```python
from build123d import *

# Parameters (mm, degrees)
SKETCH1_W           = 55.5
SKETCH1_H           = 55.5
SKETCH1_R           = 1.5
SKETCH1_W_2         = 34.5
SKETCH1_H_2         = 34.5
BOSS_EXTRUDE2_DEPTH = 2
SKETCH2_W           = 67.5
SKETCH2_H           = 67.5
SKETCH2_R           = 1.5
SKETCH2_W_2         = 55.5
SKETCH2_H_2         = 55.5
BOSS_EXTRUDE5_DEPTH = 2
SKETCH3_W           = 7
SKETCH3_H           = 7
SKETCH3_R           = 1.5
BOSS_EXTRUDE6_DEPTH = 25


with BuildPart() as part:
    # Sketch1 → Boss-Extrude2 (new body)
    with BuildSketch(Plane(origin=(0, 0, 0), x_dir=(1, 0, 0), z_dir=(0, 1, 0))):
        Rectangle(SKETCH1_W, SKETCH1_H)
        with Locations(Location((21.5, -21.5, 0), (0, 0, 270))):
            Circle(SKETCH1_R, mode=Mode.SUBTRACT)
        with Locations(Location((-21.5, -21.5, 0), (0, 0, 270))):
            Circle(SKETCH1_R, mode=Mode.SUBTRACT)
        with Locations(Location((21.5, 21.5, 0), (0, 0, 270))):
            Circle(SKETCH1_R, mode=Mode.SUBTRACT)
        with Locations(Location((-21.5, 21.5, 0), (0, 0, 270))):
            Circle(SKETCH1_R, mode=Mode.SUBTRACT)
        Rectangle(SKETCH1_W_2, SKETCH1_H_2, mode=Mode.SUBTRACT)
    extrude(amount=BOSS_EXTRUDE2_DEPTH)

    # Sketch2 → Boss-Extrude5 (add)
    with BuildSketch(Plane(origin=(0, 0, 0), x_dir=(1, 0, 0), z_dir=(0, 1, 0))):
        Rectangle(SKETCH2_W, SKETCH2_H)
        with Locations(Location((-30.25, 30.25, 0), (0, 0, 270))):
            Circle(SKETCH2_R, mode=Mode.SUBTRACT)
        with Locations(Location((30.25, 30.25, 0), (0, 0, 90))):
            Circle(SKETCH2_R, mode=Mode.SUBTRACT)
        with Locations(Location((30.25, -30.25, 0), (0, 0, 270))):
            Circle(SKETCH2_R, mode=Mode.SUBTRACT)
        with Locations(Location((-30.25, -30.25, 0), (0, 0, 90))):
            Circle(SKETCH2_R, mode=Mode.SUBTRACT)
        Rectangle(SKETCH2_W_2, SKETCH2_H_2, mode=Mode.SUBTRACT)
    extrude(amount=BOSS_EXTRUDE5_DEPTH)

    # Sketch3 → Boss-Extrude6 (add)
    # profile 1 of 4: a face of its own
    with BuildSketch(Plane(origin=(0, 0, 0), x_dir=(1, 0, 0), z_dir=(0, 1, 0))):
        with Locations((-30.25, -30.25)):
            Rectangle(SKETCH3_W, SKETCH3_H)
        with Locations(Location((-30.25, -30.25, 0), (0, 0, 90))):
            Circle(SKETCH3_R, mode=Mode.SUBTRACT)
    # profile 2 of 4: a face of its own
    with BuildSketch(Plane(origin=(0, 0, 0), x_dir=(1, 0, 0), z_dir=(0, 1, 0))):
        with Locations((30.25, -30.25)):
            Rectangle(SKETCH3_W, SKETCH3_H)
        with Locations(Location((30.25, -30.25, 0), (0, 0, 270))):
            Circle(SKETCH3_R, mode=Mode.SUBTRACT)
    # profile 3 of 4: a face of its own
    with BuildSketch(Plane(origin=(0, 0, 0), x_dir=(1, 0, 0), z_dir=(0, 1, 0))):
        with Locations((-30.25, 30.25)):
            Rectangle(SKETCH3_W, SKETCH3_H)
        with Locations(Location((-30.25, 30.25, 0), (0, 0, 270))):
            Circle(SKETCH3_R, mode=Mode.SUBTRACT)
    # profile 4 of 4: a face of its own
    with BuildSketch(Plane(origin=(0, 0, 0), x_dir=(1, 0, 0), z_dir=(0, 1, 0))):
        with Locations((30.25, 30.25)):
            Rectangle(SKETCH3_W, SKETCH3_H)
        with Locations(Location((30.25, 30.25, 0), (0, 0, 90))):
            Circle(SKETCH3_R, mode=Mode.SUBTRACT)
    extrude(amount=BOSS_EXTRUDE6_DEPTH)


solid = part.part
```
Geometry check sheet. Reference: the model listing, model coordinates, mm. A direction names the side the tool comes from. Round coordinates to 2 decimals unless told otherwise and drop trailing zeros. Loops run counter-clockwise (first coordinate to the right, second up) from the corner with the lowest first, then second, coordinate; pieces in that order, holes last. Notation, with made-up numbers: (39.25, 58.5) - (75.25, 58.5) arc R12 ccw to (75.25, 81.5) - close; hole circle Ø6 at (41.25, -3.5). An arc over 180 degrees is marked (long way). Write item = value, one per line. Start each with the question number.
1. Section check D-D on z = -5.5. Enter the section's corners in (x, y).
2. Set-up check for faces 1 (the face through (30, 13, 26.75)), 2 (the face through (26.75, 13, 30)), 3 (the face through (-30.3, 25, 28.6)), 4 (the face through (-17.25, 1, 0)): record each of +Z, -Z, +X, -X, +Y, -Y from which the full face is reachable in a straight line by a thin tool's end or side.
3. Thickness scan on line 1 (X direction, y = 8.75, z = 30.25); line 2 (X direction, y = 0.85, z = -21.5); line 3 (X direction, y = 14.25, z = 28.5). Record the ranges inside material, lowest first.
4. Depth check by flat-ended pin: pin 1 (3 mm diameter, centred on x = -25, y = 22, fed in from +Z); pin 2 (3 mm diameter, centred on x = -24.5, z = -4.5, fed in from +Y). Enter the tip coordinate at first touch or a pass-through.
5. Section check C-C on x = 9.5. Enter the section's corners in (y, z), then the cut area to 3 significant figures.
6. Section check B-B on z = -21.5. Enter the section's corners in (x, y).
7. Section check A-A on y = 21.75. Enter the section's corners in (x, z), then the cut area to 3 significant figures.
8. Mould release check, pull along X, two halves, no side actions. Record for faces 5 (the face through (0, 0, -23)), 6 (the face through (-33.75, 0.4, 0.2)), 7 (the face through (-20.49, 0.99, 20.39)): released by +X, released by -X, zero draft, split by the parting line, or undercut.
Working result:
q1.outline = (-33.75, 0) - (-17.25, 0) - (-17.25, 2) - (-33.75, 2) - close; (17.25, 0) - (33.75, 0) - (33.75, 2) - (17.25, 2) - close
q2.face_1 = +X, -X, +Y
q2.face_2 = +Z, -Z, +Y
q2.face_3 = +Z, -Z, +X, -X, +Y
q2.face_4 = +Y, -Y
q3.line_1 = -33.75 to -31.75, -28.75 to -26.75, 26.75 to 28.75, 31.75 to 33.75
q3.line_2 = -33.75 to -23, -20 to 20, 23 to 33.75
q3.line_3 = -33.75 to -26.75, 26.75 to 33.75
q4.pin_1 = through
q4.pin_2 = 2
q5.outline = (0, -33.75) - (2, -33.75) - (2, -17.25) - (0, -17.25) - close; (0, 17.25) - (2, 17.25) - (2, 33.75) - (0, 33.75) - close
q5.area = 66.0 mm^2
q6.outline = (-33.75, 0) - (-23, 0) - (-23, 2) - (-33.75, 2) - close; (-20, 0) - (20, 0) - (20, 2) - (-20, 2) - close; (23, 0) - (33.75, 0) - (33.75, 2) - (23, 2) - close
q7.outline = (-33.75, -33.75) - (-26.75, -33.75) - (-26.75, -26.75) - (-33.75, -26.75) - close; (-33.75, 26.75) - (-26.75, 26.75) - (-26.75, 33.75) - (-33.75, 33.75) - close; (26.75, -33.75) - (33.75, -33.75) - (33.75, -26.75) - (26.75, -26.75) - close; (26.75, 26.75) - (33.75, 26.75) - (33.75, 33.75) - (26.75, 33.75) - close; hole circle Ø3 at (-30.25, -30.25); hole circle Ø3 at (-30.25, 30.25); hole circle Ø3 at (30.25, -30.25); hole circle Ø3 at (30.25, 30.25)
q7.area = 168 mm^2
q8.face_5 = zero draft
q8.face_6 = released by -X
q8.face_7 = undercut
